Job drawing, mm, ordinate dimensions from the low corner. One solid piece. A direction names the side the tool comes from. Coordinates: 2 decimals unless noted, no trailing zeros. Loops run counter-clockwise (first coordinate to the right, second up) from the corner with the lowest first, then second, coordinate; pieces in that order, holes last. Notation, with made-up numbers: (-39, -35) -> (-23, -35) arc R21 cw to (-23, -8) -> close; hole circle Ø4 at (-30, 38). An arc over 180 degrees is marked (long way). Answer as CSV lines item,"result". Start each with the question number.
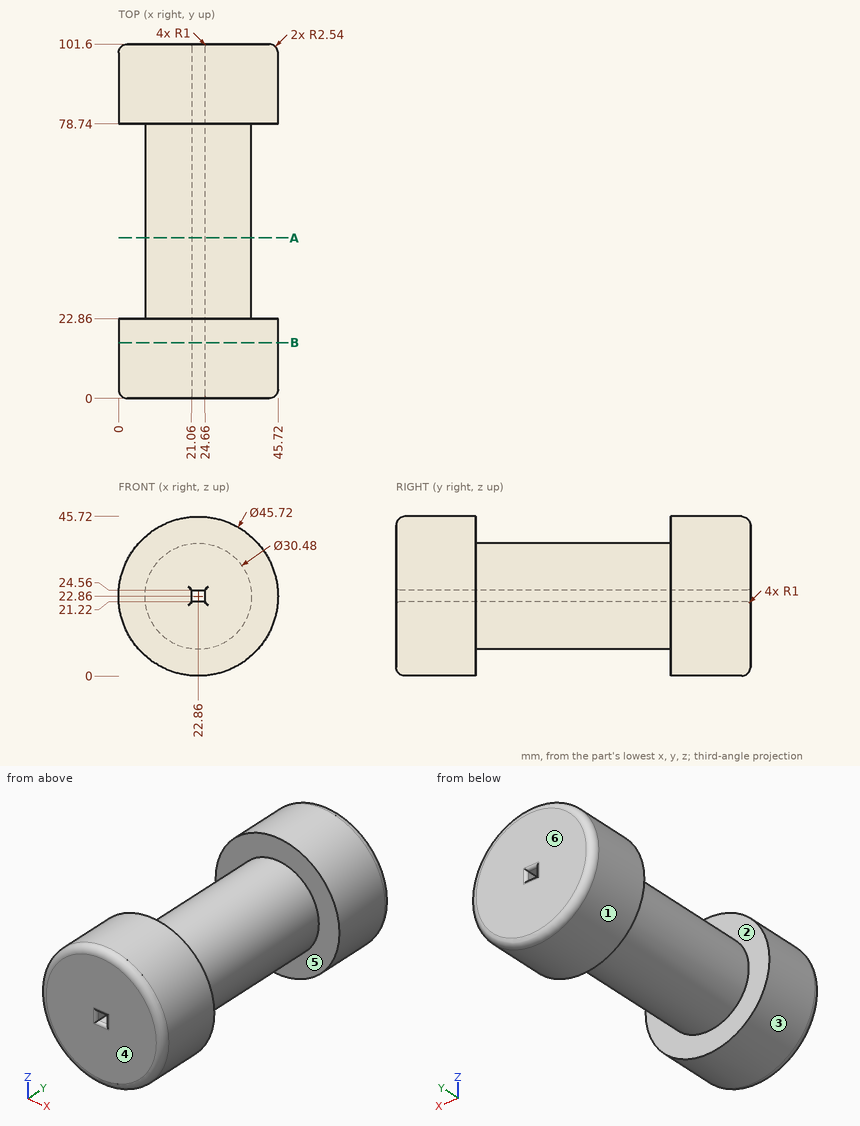
Item 1: Saw through at A-A (y = 46). Write the cut outline in (x, z).
Item 2: Wall check: probe 1 along Y at (x, z) = (15.5, 37); probe 2 along Y at (x, z) = (39.5, 8); probe 3 along X at (y, z) = (91, 13). Give the ranges that are in metal, low to high.
Item 3: Saw through at B-B (y = 16). Write the cut outline in (x, z).
Item 4: Flat gauge pins, fed straight in: pin 1 Ø1 at (y, z) = (74, 15.5) entering from +X; pin 2 Ø1.7 at (y, z) = (45.5, 23) entering from +X; pin 3 Ø3 at (x, y) = (22, 73) entering from -Z. Where does each tip first touch, or does it go through?
Item 5: Which spindle directions (+Z, -Z, +X, -X, +Y, -Y) get a long thin tool onto all of the face, cutting with end or side? Do the marked faces 1 and 2. Say none if no direction does.
Item 6: Two-plate mould, pull along Y, no slides. Class the marked faces 3, 4, 5 and 6: pulls with the +Y half, pulls with the -Y half, needs draft (parallel to the pull), parting line crosses it, or undercut.
Geometry check:
1,outline,"circle Ø30.48 at (22.86, 22.86); hole (21.06, 21.22) -> (24.66, 21.22) -> (24.66, 24.56) -> (21.06, 24.56) -> close"
2,probe 1,"0 to 22.86, 78.74 to 101.6"
2,probe 2,"0.96 to 22.86, 78.74 to 100.64"
2,probe 3,"2.24 to 43.48"
3,outline,"circle Ø45.72 at (22.86, 22.86); hole (21.06, 21.22) -> (24.66, 21.22) -> (24.66, 24.56) -> (21.06, 24.56) -> close"
4,pin 1,"x = 36.47"
4,pin 2,"x = 38.1"
4,pin 3,"z = 7.62"
5,face 1,"+Y, -Y"
5,face 2,"none"
6,face 3,"needs draft"
6,face 4,"pulls with the -Y half"
6,face 5,"undercut"
6,face 6,"pulls with the +Y half"
